Autodesk Inventor part; units mm, degrees
ref_plane "YZ Plane" through (0, 0, 0) normal (1, 0, 0) x (0, 1, 0)
ref_plane "XZ Plane" through (0, 0, 0) normal (0, 1, 0) x (-1, 0, 0)
ref_plane "XY Plane" through (0, 0, 0) normal (0, 0, 1) x (1, 0, 0)
sketch "Sketch1" plane through (0, 0, 0) normal (0, 1, 0) x (-1, 0, 0)
  line L0 (-18.75, 52.5) -> (26.25, 52.5)
  line L1 (26.25, 52.5) -> (26.25, -37.5)
  line L2 (26.25, -37.5) -> (-18.75, -37.5)
  line L3 (-18.75, -37.5) -> (-18.75, 52.5)
  line L4 (26.25, 52.5) -> (-18.75, -37.5) construction
  line L5 (-16.4706, 50) -> (23.5294, 50)
  line L6 (23.5294, 50) -> (23.5294, -35)
  line L7 (23.5294, -35) -> (-16.4706, -35)
  line L8 (-16.4706, -35) -> (-16.4706, 50)
  line L9 (23.5294, 50) -> (-16.4706, -35) construction
  line L10 (23.5294, 50) -> (21.0294, 50)
  line L11 (21.0294, 50) -> (21.0294, 47.5)
  line L12 (21.0294, 47.5) -> (23.5294, 47.5)
  line L13 (23.5294, 47.5) -> (23.5294, 50)
  arc A0 (23.5294, 47.5) -> (21.0294, 50) centre (21.0294, 47.5) ccw
  line L14 (26.25, 52.5) -> (22.75, 52.5)
  line L15 (22.75, 52.5) -> (22.75, 49)
  line L16 (22.75, 49) -> (26.25, 49)
  line L17 (26.25, 49) -> (26.25, 52.5)
  line L18 (23.5294, -35) -> (21.0294, -35)
  line L19 (21.0294, -35) -> (21.0294, -32.5)
  line L20 (21.0294, -32.5) -> (23.5294, -32.5)
  line L21 (23.5294, -32.5) -> (23.5294, -35)
  line L22 (-16.4706, -35) -> (-13.9706, -35)
  line L23 (-13.9706, -35) -> (-13.9706, -32.5)
  line L24 (-13.9706, -32.5) -> (-16.4706, -32.5)
  line L25 (-16.4706, -32.5) -> (-16.4706, -35)
  line L26 (-16.4706, 50) -> (-13.9706, 50)
  line L27 (-13.9706, 50) -> (-13.9706, 47.5)
  line L28 (-13.9706, 47.5) -> (-16.4706, 47.5)
  line L29 (-16.4706, 47.5) -> (-16.4706, 50)
  arc A1 (-13.9706, 50) -> (-16.4706, 47.5) centre (-13.9706, 47.5) ccw
  arc A2 (-16.4706, -32.5) -> (-13.9706, -35) centre (-13.9706, -32.5) ccw
  arc A3 (21.0294, -35) -> (23.5294, -32.5) centre (21.0294, -32.5) ccw
  arc A4 (26.25, 49) -> (22.75, 52.5) centre (22.75, 49) ccw
  line L30 (26.25, -37.5) -> (22.75, -37.5)
  line L31 (22.75, -37.5) -> (22.75, -34)
  line L32 (22.75, -34) -> (26.25, -34)
  line L33 (26.25, -34) -> (26.25, -37.5)
  line L34 (-18.75, -37.5) -> (-15.25, -37.5)
  line L35 (-15.25, -37.5) -> (-15.25, -34)
  line L36 (-15.25, -34) -> (-18.75, -34)
  line L37 (-18.75, -34) -> (-18.75, -37.5)
  line L38 (-18.75, 52.5) -> (-15.25, 52.5)
  line L39 (-15.25, 52.5) -> (-15.25, 49)
  line L40 (-15.25, 49) -> (-18.75, 49)
  line L41 (-18.75, 49) -> (-18.75, 52.5)
  arc A5 (-15.25, 52.5) -> (-18.75, 49) centre (-15.25, 49) ccw
  arc A6 (-18.75, -34) -> (-15.25, -37.5) centre (-15.25, -34) ccw
  arc A7 (22.75, -37.5) -> (26.25, -34) centre (22.75, -34) ccw
  point P0 (0, 0)
  point P1 (26.25, 49)
  point P2 (22.75, 52.5)
  point P3 (-18.75, -34)
  point P4 (-16.4706, -32.5)
  point P5 (-15.9706, -34)
  point P6 (-16.4706, -34)
  point P7 (23.5294, -32.5)
  dimension "d0" = 45
  dimension "d1" = 90
  dimension "d2" = 40
  dimension "d3" = 85
  dimension "d8" = 2.5
  dimension "d9" = 2.5
extrude "Extrusion3" add sketch "Sketch1" along normal blind 2.5 contours L0 L15 L5 L39 | L39 L5 L8 L40 A5 | L40 L8 L36 L3 | A4 L16 L6 L5 L15 | L39 A1 L40 L8 L5 | L5 A1 L39 | L36 L8 L7 L35 A6 | L40 A1 L8 | L15 A0 L5 | L5 L6 L16 A0 L15 | L1 L32 L6 L16 | L5 L11 L12 L6 L20 L19 L7 L23 L24 L8 L28 L27 | L27 L28 A1 L40 L39 | L39 L40 A1 | L36 A2 L35 L7 L8 | L35 L7 L31 L2 | A0 L15 L16 L12 L11 | A0 L16 L15 | A7 L31 L7 L6 L32 | L6 A0 L16 | L24 L23 A2 L35 L36 | L36 L35 A2 | L35 A2 L7 | L32 A3 L6 | L6 L7 L31 A3 L32 | L7 A3 L31 | A3 L32 L31 L19 L20 | A3 L31 L32
fillet "Fillet1" radius 3 8 edges at (-25.2249, 0, 51.4749) (-3.75, 0, 52.5) (17.7249, 0, 51.4749) (18.75, 0, 7.5) (17.7249, 0, -36.4749) (-3.75, 0, -37.5) (-25.2249, 0, -36.4749) (-26.25, 0, 7.5)
sketch "Sketch2" plane through (0, 2.5, 0) normal (0, 1, 0) x (1, 0, 0)
  arc A0 (16.4706, 32.5) -> (13.9706, 35) centre (13.9706, 32.5) ccw
  line L0 (13.9706, 35) -> (13.9706, 33.5)
  line L1 (16.4706, -47.5) -> (16.4706, 32.5)
  line L2 (16.4706, 32.5) -> (14.9706, 32.5)
  line L3 (14.9706, 32.5) -> (13.9706, 33.5)
  line L4 (14.4706, 33) -> (12.526, 31.0555)
  circle A1 centre (12.526, 31.0555) radius 2.75
  line L5 (-23.5294, 32.5) -> (-23.5294, -47.5)
  line L6 (-23.5294, -47.5) -> (-22.0294, -47.5)
  line L7 (-21.0294, -50) -> (13.9706, -50)
  line L8 (-21.0294, -50) -> (-21.0294, -48.5)
  line L9 (-21.0294, -48.5) -> (-22.0294, -47.5)
  line L10 (-21.5294, -48) -> (-19.5849, -46.0555)
  line L11 (-21.5294, -48) -> (-18.7794, -48) construction
  circle A2 centre (-19.5849, -46.0555) radius 2.75
  arc A3 (14.0518, 28.7675) -> (15.276, 31.0555) centre (12.526, 31.0555) ccw construction
  arc A4 (14.321, 28.3639) -> (15.7612, 31.0555) centre (12.526, 31.0555) ccw
  arc A5 (13.7826, 29.1712) -> (14.7909, 31.0555) centre (12.526, 31.0555) ccw
  arc A6 (13.7826, 29.1712) -> (14.321, 28.3639) centre (14.0518, 28.7675) ccw
  arc A7 (15.7612, 31.0555) -> (14.7909, 31.0555) centre (15.276, 31.0555) ccw
  arc A8 (10.7311, 33.747) -> (9.2909, 31.0555) centre (12.526, 31.0555) ccw
  arc A9 (9.2909, 31.0555) -> (10.2612, 31.0555) centre (9.776, 31.0555) ccw
  arc A10 (11.2694, 32.9398) -> (10.7311, 33.747) centre (11.0003, 33.3434) ccw
  arc A11 (11.2694, 32.9398) -> (10.2612, 31.0555) centre (12.526, 31.0555) ccw
  arc A12 (-17.79, -48.747) -> (-16.3497, -46.0555) centre (-19.5849, -46.0555) ccw
  arc A13 (-18.3283, -47.9398) -> (-17.32, -46.0555) centre (-19.5849, -46.0555) ccw
  arc A14 (-18.3283, -47.9398) -> (-17.79, -48.747) centre (-18.0591, -48.3434) ccw
  arc A15 (-16.3497, -46.0555) -> (-17.32, -46.0555) centre (-16.8349, -46.0555) ccw
  arc A16 (-21.3798, -43.3639) -> (-22.82, -46.0555) centre (-19.5849, -46.0555) ccw
  arc A17 (-22.82, -46.0555) -> (-21.8497, -46.0555) centre (-22.3349, -46.0555) ccw
  arc A18 (-20.8415, -44.1712) -> (-21.3798, -43.3639) centre (-21.1106, -43.7675) ccw
  arc A19 (-20.8415, -44.1712) -> (-21.8497, -46.0555) centre (-19.5849, -46.0555) ccw
  line L12 (-22.8137, -49.2843) -> (-20.2452, -46.7157) construction
  line L13 (-22.3894, -49.7085) -> (-19.8209, -47.14)
  line L14 (-20.6694, -46.2915) -> (-23.2379, -48.86)
  arc A20 (-23.2379, -48.86) -> (-22.3894, -49.7085) centre (-22.8137, -49.2843) ccw
  arc A21 (-19.8209, -47.14) -> (-20.6694, -46.2915) centre (-20.2452, -46.7157) ccw
  line L15 (12.9911, 31.5205) -> (15.9501, 34.4795) construction
  line L16 (13.4153, 31.0962) -> (16.3744, 34.0552)
  line L17 (15.5258, 34.9038) -> (12.5668, 31.9448)
  arc A22 (12.5668, 31.9448) -> (13.4153, 31.0962) centre (12.9911, 31.5205) ccw
  arc A23 (16.3744, 34.0552) -> (15.5258, 34.9038) centre (15.9501, 34.4795) ccw
  arc A24 (15.25, -52.5) -> (18.75, -49) centre (15.25, -49) ccw
  line L18 (15.25, -52.5) -> (18.75, -52.5)
  line L19 (18.75, -52.5) -> (18.75, -49)
  arc A25 (-22.75, 37.5) -> (-26.25, 34) centre (-22.75, 34) ccw
  line L20 (-26.25, 34) -> (-26.25, 37.5)
  line L21 (15.25, 37.5) -> (-22.75, 37.5)
  line L22 (-26.25, 37.5) -> (-22.75, 37.5)
  line L23 (-22.75, -52.5) -> (15.25, -52.5)
  line L24 (-22.75, -52.5) -> (-26.25, -52.5)
  line L25 (-26.25, 34) -> (-26.25, -49)
  line L26 (-26.25, -52.5) -> (-26.25, -49)
  line L27 (18.75, -49) -> (18.75, 34)
  line L28 (18.75, 37.5) -> (18.75, 34)
  line L29 (15.25, 37.5) -> (15.25, 34.542)
  line L30 (18.75, 37.5) -> (15.25, 37.5)
  line L31 (-26.25, -52.5) -> (18.75, 37.5)
  line L32 (18.75, -52.5) -> (-26.25, 37.5)
  line L33 (-3.75, -7.5) -> (32.3445, -7.5)
  line L34 (-35.1724, -7.5) -> (-3.75, -7.5)
  circle A26 centre (12.526, -46.0555) radius 2.75
  circle A27 centre (-19.5849, 31.0555) radius 2.75
  point P0 (0, 0)
  point P1 (14.848, 32.5289)
  point P2 (13.9995, 33.3774)
  point P3 (11.4261, 33.5759)
  point P4 (9.8188, 30.5722)
  point P5 (13.626, 28.535)
  point P6 (15.2333, 31.5387)
  point P7 (-21.9068, -47.5289)
  point P8 (-21.0583, -48.3774)
  point P9 (-18.4849, -48.5759)
  point P10 (-16.8777, -45.5722)
  point P11 (-20.6848, -43.535)
  point P12 (-22.2921, -46.5387)
  point P13 (15.2624, 34.6404)
  point P14 (16.111, 33.7918)
  point P15 (14.6612, -44.3223)
  point P16 (15.1936, -45.3873)
  dimension "d32" = 5.5
  dimension "d29" = 1.5
  dimension "d30" = 1.5
  dimension "d31" = 2.75
  dimension "d33" = 1.5
  dimension "d34" = 1.5
  dimension "d35" = 2.75
  dimension "d36" = 45
  dimension "d37" = 5.5
  dimension "d40" = 360
  dimension "d44" = 1.2
  dimension "d45" = 1.2
extrude "Extrusion10" cut sketch "Sketch2" against normal blind 10 contours L32 A26 | A27 picked at (11.7147, -45.435)
sketch "Sketch4" plane through (0, 2.5, 0) normal (0, 1, 0) x (1, 0, 0)
  point P0 (0, 0)
properties part number "proper shit spodnji"
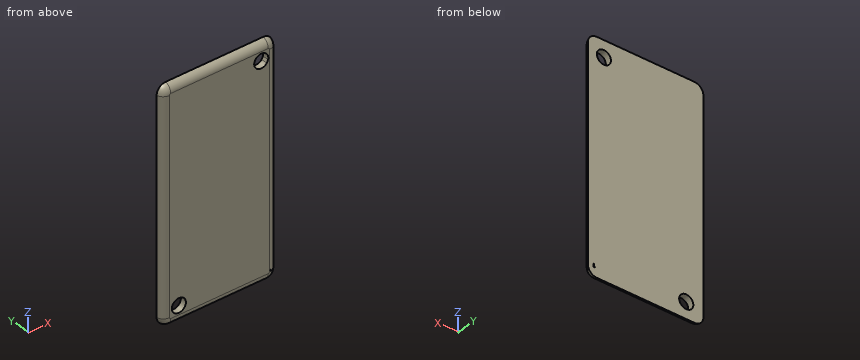
Design review of the part built by this model. Coordinates are the model's own, in mm. Coordinates: 2 decimals unless noted, no trailing zeros. Loops run counter-clockwise (first coordinate to the right, second up) from the corner with the lowest first, then second, coordinate; pieces in that order, holes last. Notation, with made-up numbers: (9, -4.75) -> (29, -4.75) arc R8 ccw to (29, 9.25) -> close; hole circle Ø5 at (-4, -38.5). An arc over 180 degrees is marked (long way). Use a Markdown table: item, result. Add a question column.
Item 1: We need section C-C, the plane x = -11. Write out the cut boundary in (y, z).
Item 2: Wall thickness on L1, parallel to Z at x = 14, y = 2.25; L2, parallel to Z at x = -17.5, y = 2; L3, parallel to Z at x = -10, y = 2.4: over which ranges is each line inside the solid? List them lowest first. Write a range as from..to.
Item 3: We need section A-A, the plane x = -20.5. Write out the cut boundary in (y, z), and give its area (3 significant figures).
Item 4: We need section D-D, the plane y = 0.6. Count the separate pieces of the cut face and the enclosed holes in it, and give its area (3 significant figures).
Item 5: We need section B-B, the plane z = -9.5. Write out the cut boundary in (x, y), and give its area (3 significant figures).
Item 6: Clearance check with flat-ended pins moving along their axes: P1, Ø1.5, axis at x = 13, y = 0.5, coming from the +Z side; P2, Ø0.8, axis at y = 1.5, z = -33, coming from the -X side; P3, Ø0.6, axis at x = 16.5, y = 1, coming from the +Z side. State where each tip first meets the part, or that it passes through.
Numbers:
| question | item | result |
|---|---|---|
| 1 | outline | (0, -34.54) arc R3 ccw to (2.5, -37.5) -> (2.5, 52.5) arc R3 ccw to (0, 49.54) -> close |
| 2 | L1 | z = -37.45..43.73, 48.38..52.45 |
| 2 | L2 | z = -37.37..-32.85, -29.26..52.37 |
| 2 | L3 | z = -37.48..52.48 |
| 3 | outline | (0, -34.54) arc R3 ccw to (2.5, -37.5) -> (2.5, -33.65) -> (0, -33.65) -> close; (0, -28.46) -> (2.5, -28.46) -> (2.5, 52.5) arc R3 ccw to (0, 49.54) -> close |
| 3 | area | 208 mm^2 |
| 4 | separate pieces | 1 |
| 4 | enclosed holes | 3 |
| 4 | area | 3,690 mm^2 |
| 5 | outline | (-26.25, 2.5) arc R3 ccw to (-23.29, 0) -> (15.79, 0) arc R3 ccw to (18.75, 2.5) -> close |
| 5 | area | 109 mm^2 |
| 6 | P1 | stops at z = 51.98 |
| 6 | P2 | stops at x = -26.08 |
| 6 | P3 | stops at z = 51.78 |
